```python
from build123d import *

# Parameters (mm, degrees)
SKETCH2_W           = 124
SKETCH2_H           = 42.5
SKETCH2_R           = 12.5
SKETCH2_R_2         = 6
SKETCH2_R_3         = 1.5
BOSS_EXTRUDE1_DEPTH = 50
SKETCH3_W           = 42.5
SKETCH3_H           = 42.5
CUT_EXTRUDE1_DEPTH  = 39
SKETCH4_W           = 33.75
SKETCH4_H           = 42.5
CUT_EXTRUDE2_DEPTH  = 30
CUT_EXTRUDE3_REACH  = 44.5
SKETCH5_R           = 2.1
CUT_EXTRUDE4_DEPTH  = 3


with BuildPart() as part:
    # Sketch2 → Boss-Extrude1 (new body)
    with BuildSketch(Plane.XY):
        with Locations((62, 21.25)):
            Rectangle(SKETCH2_W, SKETCH2_H)
        with Locations((62, 21.25)):
            Circle(SKETCH2_R, mode=Mode.SUBTRACT)
        with Locations((107, 21.25)):
            Circle(SKETCH2_R_2, mode=Mode.SUBTRACT)
        with Locations((17, 21.25)):
            Circle(SKETCH2_R_2, mode=Mode.SUBTRACT)
        with Locations((46.5, 36.75)):
            Circle(SKETCH2_R_3, mode=Mode.SUBTRACT)
        with Locations((77.5, 36.75)):
            Circle(SKETCH2_R_3, mode=Mode.SUBTRACT)
        with Locations((77.5, 5.75)):
            Circle(SKETCH2_R_3, mode=Mode.SUBTRACT)
        with Locations((46.5, 5.75)):
            Circle(SKETCH2_R_3, mode=Mode.SUBTRACT)
    extrude(amount=BOSS_EXTRUDE1_DEPTH)

    # Sketch3 → Cut-Extrude1 (cut)
    with BuildSketch(Plane.XY.offset(50)):
        with Locations((62, 21.25)):
            Rectangle(SKETCH3_W, SKETCH3_H)
    extrude(amount=-CUT_EXTRUDE1_DEPTH, mode=Mode.SUBTRACT)

    # Sketch4 → Cut-Extrude2 (cut)
    with BuildSketch(Plane(origin=(0, 0, 0), x_dir=(-1, 0, 0), z_dir=(0, 0, -1))):
        with Locations((-107.125, 21.25)):
            Rectangle(SKETCH4_W, SKETCH4_H)
        with Locations((-16.875, 21.25)):
            Rectangle(SKETCH4_W, SKETCH4_H)
    extrude(amount=-CUT_EXTRUDE2_DEPTH, mode=Mode.SUBTRACT)

    # Sketch5 → Cut-Extrude3 (cut, up to next)
    with BuildSketch(Plane.XZ, mode=Mode.PRIVATE) as cut_extrude3_sk1:
        with Locations((7, 40)):
            Circle(SKETCH5_R)
    cut_extrude3_tool1 = extrude(cut_extrude3_sk1.sketch, amount=-CUT_EXTRUDE3_REACH, mode=Mode.PRIVATE) & part.part
    add(cut_extrude3_tool1.solids().sort_by_distance((7, 0, 40))[0], mode=Mode.SUBTRACT)
    # Sketch5 → Cut-Extrude3 (cut, up to next)
    with BuildSketch(Plane.XZ, mode=Mode.PRIVATE) as cut_extrude3_sk2:
        with Locations((27, 40)):
            Circle(SKETCH5_R)
    cut_extrude3_tool2 = extrude(cut_extrude3_sk2.sketch, amount=-CUT_EXTRUDE3_REACH, mode=Mode.PRIVATE) & part.part
    add(cut_extrude3_tool2.solids().sort_by_distance((27, 0, 40))[0], mode=Mode.SUBTRACT)
    # Sketch5 → Cut-Extrude3 (cut, up to next)
    with BuildSketch(Plane.XZ, mode=Mode.PRIVATE) as cut_extrude3_sk3:
        with Locations((97, 40)):
            Circle(SKETCH5_R)
    cut_extrude3_tool3 = extrude(cut_extrude3_sk3.sketch, amount=-CUT_EXTRUDE3_REACH, mode=Mode.PRIVATE) & part.part
    add(cut_extrude3_tool3.solids().sort_by_distance((97, 0, 40))[0], mode=Mode.SUBTRACT)
    # Sketch5 → Cut-Extrude3 (cut, up to next)
    with BuildSketch(Plane.XZ, mode=Mode.PRIVATE) as cut_extrude3_sk4:
        with Locations((117, 40)):
            Circle(SKETCH5_R)
    cut_extrude3_tool4 = extrude(cut_extrude3_sk4.sketch, amount=-CUT_EXTRUDE3_REACH, mode=Mode.PRIVATE) & part.part
    add(cut_extrude3_tool4.solids().sort_by_distance((117, 0, 40))[0], mode=Mode.SUBTRACT)
    # Sketch5 → Cut-Extrude3 (cut, up to next)
    with BuildSketch(Plane.XZ, mode=Mode.PRIVATE) as cut_extrude3_sk5:
        with Locations((17, 40)):
            Circle(SKETCH5_R)
    cut_extrude3_tool5 = extrude(cut_extrude3_sk5.sketch, amount=-CUT_EXTRUDE3_REACH, mode=Mode.PRIVATE) & part.part
    add(cut_extrude3_tool5.solids().sort_by_distance((17, 0, 40))[0], mode=Mode.SUBTRACT)
    # Sketch5 → Cut-Extrude3 (cut, up to next)
    with BuildSketch(Plane.XZ, mode=Mode.PRIVATE) as cut_extrude3_sk6:
        with Locations((107, 40)):
            Circle(SKETCH5_R)
    cut_extrude3_tool6 = extrude(cut_extrude3_sk6.sketch, amount=-CUT_EXTRUDE3_REACH, mode=Mode.PRIVATE) & part.part
    add(cut_extrude3_tool6.solids().sort_by_distance((107, 0, 40))[0], mode=Mode.SUBTRACT)

    # Sketch7 → Cut-Extrude4 (cut)
    with BuildSketch(Plane.XY.offset(50)):
        Polygon((0, 40.5), (40.75, 22.5), (40.75, 18.5), (0, 36.5), align=None)
    extrude(amount=-CUT_EXTRUDE4_DEPTH, mode=Mode.SUBTRACT)


solid = part.part
```
Design review of the part built by this model. Coordinates are the model's own, in mm. A direction names the side the tool comes from. Coordinates: 2 decimals unless noted, no trailing zeros. Write each loop counter-clockwise with the first axis right and the second up, starting at its lowest first coordinate (ties: lowest second). Pieces come first, ordered by that corner, then holes.
1) To check wall thickness, follow L1, parallel to X at y = 28, z = 19; L2, parallel to X at y = 36.75, z = 6.25; L3, parallel to X at y = 4.5, z = 37.5. State the ranges of each line that lie inside material, in increasing order.
2) Add section A-A (x = 69.5). Write out the cut boundary in (y, z).
3) Insertion check: pin 1 (3.5 mm diameter, centred on x = 27, z = 40, fed in from -Y); pin 2 (3.5 mm diameter, centred on x = 46.5, y = 36.75, fed in from -Z); pin 3 (3.5 mm diameter, centred on x = 107, z = 40, fed in from -Y); pin 4 (4 mm diameter, centred on x = 111.5, y = 18.5, fed in from -Z). Each pin has a flat end and moves straight along its axis. Give the tip position at first contact, or say it passes through.
4) Add section D-D (z = 22). Write out the cut boundary in (x, y).
5) Mouldability with a two-part tool opening along X and no side actions: class faces 6 (the flat face through (90.25, 21, 15)), 7 (the flat face through (20.66, 27.374, 48.521)), 8 (the flat face through (99, 22, 50)) as +X half, -X half, draft (parallel to the pull), parting line (faces both ways), or undercut.
6) Add section C-C (x = 46.5). Write out the cut boundary in (y, z).
7) Machinability: for faces 1 (the flat face through (20.09, 31.626, 48.521)), 2 (the cylindrical face through (17.969, 7.705, 38.137)), 3 (the flat face through (33.75, 21, 15)), 4 (the cylindrical face through (106.22, 27.2, 39.86)), 5 (the flat face through (83.25, 21, 31)), which of the approach directions +Z, -Z, +X, -X, +Y, -Y give a long, thin tool a straight path to every point of the face, cutting with its end or side? Answer none if there is none.
8) Add section B-B (y = 5.75). State how many separate pieces and enclosed holes the cut face has, plus the area to 3 significant figures.
Check result:
1. L1: x = 33.75 to 40.75, 83.25 to 90.25
1. L2: x = 33.75 to 45, 48 to 76, 79 to 90.25
1. L3: x = 0 to 40.75, 83.25 to 124
2. outline: (0, 0) - (11.25, 0) - (11.25, 11) - (0, 11) - close; (31.25, 0) - (42.5, 0) - (42.5, 11) - (31.25, 11) - close
3. pin 1: passes through
3. pin 2: stops at z = 0
3. pin 3: stops at y = 26.99
3. pin 4: stops at z = 30
4. outline: (33.75, 0) - (40.75, 0) - (40.75, 42.5) - (33.75, 42.5) - close; (83.25, 0) - (90.25, 0) - (90.25, 42.5) - (83.25, 42.5) - close
5. face 6: +X half
5. face 7: undercut
5. face 8: draft
6. outline: (0, 0) - (4.25, 0) - (4.25, 11) - (0, 11) - close; (7.25, 0) - (35.25, 0) - (35.25, 11) - (7.25, 11) - close; (38.25, 0) - (42.5, 0) - (42.5, 11) - (38.25, 11) - close
7. face 1: +Z
7. face 2: -Y
7. face 3: -Z, -X, +Y, -Y
7. face 4: +Z, -Z
7. face 5: +Z, +Y, -Y
8. separate pieces: 3
8. enclosed holes: 6
8. area: 2,370 mm2
